Autodesk Inventor part; units mm, degrees
ref_plane "YZ Plane" through (0, 0, 0) normal (1, 0, 0) x (0, 1, 0)
ref_plane "XZ Plane" through (0, 0, 0) normal (0, 1, 0) x (-1, 0, 0)
ref_plane "XY Plane" through (0, 0, 0) normal (0, 0, 1) x (1, 0, 0)
sketch "Sketch1" plane through (0, 0, 0) normal (0, 0, 1) x (1, 0, 0)
  line L0 (0, 0) -> (34.5, 0)
  line L1 (34.5, 0) -> (34.5, 15.7)
  line L2 (34.5, 15.7) -> (0, 15.7)
  line L3 (0, 15.7) -> (0, 0)
  dimension "d0" = 34.5
  dimension "d1" = 15.7
extrude "Extrusion1" add sketch "Sketch1" along normal blind 1
sketch "Sketch3" plane through (34.5, 0, 0) normal (1, 0, 0) x (0, 0, -1)
  line L0 (-1, 0) -> (-1, 15.7)
  line L1 (-1, 15.3) -> (-0.7, 15.3)
  line L2 (-0.7, 15.3) -> (-0.7, 14.8)
  line L3 (-0.7, 14.8) -> (-1, 14.8)
  line L4 (-1, 14.8) -> (-1, 15.3)
  line L5 (0, 15.7) -> (-1, 15.7)
  dimension "d8" = 0.3
  dimension "d9" = 0.5
  dimension "d12" = 0.4
extrude "Extrusion3" cut sketch "Sketch3" against normal blind 40
sketch "Sketch5" plane through (0, 0, 0) normal (0, 0, -1) x (-1, 0, 0)
  line L0 (-1.5, 13.18) -> (-3.5, 13.18)
  line L1 (-3.5, 13.18) -> (-3.5, 2.5199)
  line L2 (-3.5, 2.5199) -> (-1.5, 2.5199)
  line L3 (-1.5, 2.5199) -> (-1.5, 13.18)
  line L4 (0, 15.7) -> (0, 0)
  line L5 (-34.5, 15.7) -> (0, 15.7)
  dimension "d18" = 2
  dimension "d19" = 10.6601
  dimension "d20" = 2.52
  dimension "d21" = 1.5
extrude "Extrusion5" cut sketch "Sketch5" against normal blind 2
properties part number "Zijkant 2"
The listing builds one solid part. Answer for the finished solid, in the listing's coordinates (mm). A direction names the side the tool comes from. Round coordinates to 2 decimals unless told otherwise and drop trailing zeros. Loops run counter-clockwise (first coordinate to the right, second up) from the corner with the lowest first, then second, coordinate; pieces in that order, holes last. Notation, with made-up numbers: (20, 82.25) - (79, 82.25) arc R20 ccw to (79, 88.25) - close; hole circle Ø8 at (56.5, 84). An arc over 180 degrees is marked (long way). Use one line per item in the form item = value. Start each with the question number.
1. The part is cut by section B-B on z = 0.2. Determine the outline of the cut face in (x, y).
2. Given pin 1 Ø1.5 at (x, y) = (4, 13) entering from -Z, flat-ended and moving along its own axis, determine where the tip first touches the part or whether it passes through.
3. Consider line 1 (X direction, y = 12, z = 0.45); line 2 (Y direction, x = 21.5, z = 0.8); line 3 (Z direction, x = 26, y = 15.25). Determine where each line is inside the solid, lowest interval first. Write a range as [from, to].
4. For a pull along X with two mould halves and no side action, classify faces 3 (the face through (17, 8, 1)), 4 (the face through (2.5, 2.52, 0.5)), 5 (the face through (0, 8, 0.5)) as pulls with the +X half, pulls with the -X half, needs draft (parallel to the pull), parting line crosses it, or undercut.
5. The part is cut by section A-A on y = 8.5. Determine the outline of the cut face in (x, z).
6. A tool of negligible diameter and unlimited length cuts with its end or side. For faces 1 (the face through (17, 0, 0.5)), 2 (the face through (2.5, 13.18, 0.5)), from which of +Z, -Z, +X, -X, +Y, -Y can it reach the whole face along a straight path? Write none if from no direction.
Geometry check:
q1.outline = (0, 0) - (34.5, 0) - (34.5, 15.7) - (0, 15.7) - close; hole (1.5, 2.52) - (3.5, 2.52) - (3.5, 13.18) - (1.5, 13.18) - close
q2.pin_1 = 0
q3.line_1 = [0, 1.5], [3.5, 34.5]
q3.line_2 = [0, 14.8], [15.3, 15.7]
q3.line_3 = [0, 0.7]
q4.face_3 = needs draft
q4.face_4 = undercut
q4.face_5 = pulls with the -X half
q5.outline = (0, 0) - (1.5, 0) - (1.5, 1) - (0, 1) - close; (3.5, 0) - (34.5, 0) - (34.5, 1) - (3.5, 1) - close
q6.face_1 = +Z, -Z, +X, -X, -Y
q6.face_2 = +Z, -Z
